from build123d import *

# Parameters (mm, degrees)
SKETCH_2_R      = 1.75
SKETCH_2_R_2    = 1.5
EXTRUDE_2_DEPTH = 3


with BuildPart() as part:
    # 草图2 → 凸台-拉伸2 (new body)
    with BuildSketch(Plane.XY):
        with BuildLine():
            Line((-73, 0), (73, 0))
            ThreePointArc((73, 0), (77.949747468, 2.050252532), (80, 7))
            Line((80, 7), (80, 60))
            Line((80, 60), (105, 60))
            ThreePointArc((105, 60), (110.7284389, 62.976942983), (111.584524662, 69.375717782))
            Line((111.584524662, 69.375717782), (76.947414353, 165.375717782))
            ThreePointArc((76.947414353, 165.375717782), (74.385946708, 168.7284389), (70.362889691, 170))
            Line((70.362889691, 170), (-70.362889691, 170))
            ThreePointArc((-70.362889691, 170), (-74.385946708, 168.7284389), (-76.947414353, 165.375717782))
            Line((-76.947414353, 165.375717782), (-111.584524662, 69.375717782))
            ThreePointArc((-111.584524662, 69.375717782), (-110.7284389, 62.976942983), (-105, 60))
            Line((-105, 60), (-80, 60))
            Line((-80, 60), (-80, 7))
            ThreePointArc((-80, 7), (-77.949747468, 2.050252532), (-73, 0))
        make_face()
        with Locations((-70, 10)):
            Circle(SKETCH_2_R, mode=Mode.SUBTRACT)
        with Locations((-70, 40)):
            Circle(SKETCH_2_R, mode=Mode.SUBTRACT)
        with Locations(Location((-46, 40, 0), (0, 0, 180))):
            Circle(SKETCH_2_R, mode=Mode.SUBTRACT)
        with Locations(Location((-46, 10, 0), (0, 0, 180))):
            Circle(SKETCH_2_R, mode=Mode.SUBTRACT)
        with Locations((46, 10)):
            Circle(SKETCH_2_R, mode=Mode.SUBTRACT)
        with Locations((46, 40)):
            Circle(SKETCH_2_R, mode=Mode.SUBTRACT)
        with Locations(Location((70, 40, 0), (0, 0, 180))):
            Circle(SKETCH_2_R, mode=Mode.SUBTRACT)
        with Locations(Location((70, 10, 0), (0, 0, 180))):
            Circle(SKETCH_2_R, mode=Mode.SUBTRACT)
        with Locations((-72.441382232, 165.375717782)):
            Circle(SKETCH_2_R_2, mode=Mode.SUBTRACT)
        with Locations((-106.29148568, 65.75613767)):
            Circle(SKETCH_2_R_2, mode=Mode.SUBTRACT)
        with Locations(Location((106.29148568, 65.75613767, 0), (0, 0, 180))):
            Circle(SKETCH_2_R_2, mode=Mode.SUBTRACT)
        with Locations(Location((72.441382232, 165.375717782, 0), (0, 0, 180))):
            Circle(SKETCH_2_R_2, mode=Mode.SUBTRACT)
        with Locations((-20, 165)):
            Circle(SKETCH_2_R_2, mode=Mode.SUBTRACT)
        with Locations(Location((20, 165, 0), (0, 0, 180))):
            Circle(SKETCH_2_R_2, mode=Mode.SUBTRACT)
        with Locations((-75, 3.552033702)):
            Circle(SKETCH_2_R_2, mode=Mode.SUBTRACT)
        with Locations(Location((75, 3.552033702, 0), (0, 0, 180))):
            Circle(SKETCH_2_R_2, mode=Mode.SUBTRACT)
        with BuildLine():
            Line((-11.490577198, 151.277899951), (11.509422802, 151.277899951))
            ThreePointArc((11.509422802, 151.277899951), (13.601072868, 151.971656911), (14.863524768, 153.777899951))
            ThreePointArc((14.863524768, 153.777899951), (13.601072868, 155.584142991), (11.509422802, 156.277899951))
            Line((11.509422802, 156.277899951), (-11.490577198, 156.277899951))
            ThreePointArc((-11.490577198, 156.277899951), (-13.582227264, 155.584142991), (-14.844679164, 153.777899951))
            ThreePointArc((-14.844679164, 153.777899951), (-13.582227264, 151.971656911), (-11.490577198, 151.277899951))
        make_face(mode=Mode.SUBTRACT)
        with BuildLine():
            Line((-11.5, 47.5), (11.5, 47.5))
            ThreePointArc((11.5, 47.5), (13.591650066, 48.19375696), (14.854101966, 50))
            ThreePointArc((14.854101966, 50), (13.591650066, 51.80624304), (11.5, 52.5))
            Line((11.5, 52.5), (-11.5, 52.5))
            ThreePointArc((-11.5, 52.5), (-13.591650066, 51.80624304), (-14.854101966, 50))
            ThreePointArc((-14.854101966, 50), (-13.591650066, 48.19375696), (-11.5, 47.5))
        make_face(mode=Mode.SUBTRACT)
        with BuildLine():
            Line((-10, 22.5), (10, 22.5))
            ThreePointArc((10, 22.5), (13.535533906, 23.964466094), (15, 27.5))
            Line((15, 27.5), (15, 32.5))
            ThreePointArc((15, 32.5), (13.535533906, 36.035533906), (10, 37.5))
            Line((10, 37.5), (-10, 37.5))
            ThreePointArc((-10, 37.5), (-13.535533906, 36.035533906), (-15, 32.5))
            Line((-15, 32.5), (-15, 27.5))
            ThreePointArc((-15, 27.5), (-13.535533906, 23.964466094), (-10, 22.5))
        make_face(mode=Mode.SUBTRACT)
    extrude(amount=EXTRUDE_2_DEPTH)


solid = part.part
Can you work these out from the model? Positions are in its coordinate system, mm. A direction names the side the tool comes from. Coordinates: 2 decimals unless noted, no trailing zeros. Write each loop counter-clockwise with the first axis right and the second up, starting at its lowest first coordinate (ties: lowest second). Pieces come first, ordered by that corner, then holes.
Q1. Imagine slicing it at A-A, the plane z = 2.45. Count the separate pieces of the cut face and the enclosed holes in it, plus the area to 3 significant figures.
Results found:
separate pieces: 1
enclosed holes: 19
area: 29,600 mm2
Q2. Please list where these lines run through material, in increasing order: L1, parallel to Y at x = 70, z = 1.95; L2, parallel to Y at x = -12, z = 2.65; L3, parallel to Y at x = -13, z = 2.1.
Results found:
L1: y = 0 to 8.25, 11.75 to 38.25, 41.75 to 170
L2: y = 0 to 22.92, 37.08 to 47.54, 52.46 to 151.32, 156.24 to 170
L3: y = 0 to 23.5, 36.5 to 47.84, 52.16 to 151.62, 155.94 to 170
Q3. If we mould it in two halves opening along X, with no side actions, what happens to faces 3 (the face through (-2, 86, 0)), 4 (the face through (74.435, 168.694, 1.479)), 5 (the face through (-13.5, 36.07, 1.48))? For each: +X half, -X half, draft (parallel to the pull), parting line (faces both ways), or undercut.
Results found:
face 3: draft
face 4: +X half
face 5: undercut
Q4. Imagine slicing it at C-C, the plane x = 89. List the corners of the cut face in (y, z) for me, plus the area to 3 significant figures.
Results found:
outline: (60, 0) - (131.97, 0) - (131.97, 3) - (60, 3) - close
area: 216 mm2
Q5. Which directions (+Z, -Z, +X, -X, +Y, -Y) give clear straight access to the entire face, cutting with the end or side of a thin tool? Please do faces 1 (the face through (13.57, 36, 1.48)), 2 (the face through (-110.78, 63.05, 1.48)).
Results found:
face 1: +Z, -Z
face 2: +Z, -Z, -X
Q6. Imagine slicing it at B-B, the plane y = 120.5. List the corners of the cut face in (x, z) for me, plus the area to 3 significant figures.
Results found:
outline: (-93.14, 0) - (93.14, 0) - (93.14, 3) - (-93.14, 3) - close
area: 559 mm2
Q7. For P1, Ø2.5, axis at x = 72.44, y = 165.38, coming from the +Z side; P2, Ø0.9, axis at x = -96.5, z = 2, coming from the -Y side; P3, Ø1.5, axis at y = 31, z = 1, coming from the +X side, each with a flat end and sliding along its axis, tell me the tip position at first contact or that it passes through.
Results found:
P1: passes through
P2: stops at y = 60
P3: stops at x = 80
